Verification items for this drawing (mm, ordinates from the low corner). A direction names the side the tool comes from. Round coordinates to 2 decimals unless told otherwise and drop trailing zeros. Order: outer loops, then holes, each group sorted by start corner. A loop starts at its lowest first (then second) coordinate and runs counter-clockwise, first axis right, second up. Notation, with made-up numbers: M 9.5,-29.5 L 17.5,-29.5 A31 ccw 17.5,-4.5 Z; hole C -21,85 d3. An arc over 180 degrees is marked long. One line per item, written item: value. Start each with the question number.
(1) Release check for a two-part mould opening along Z. For the marked faces 1, 2 and 3 record: released by +Z, released by -Z, zero draft, split by the parting line, or undercut.
(2) Thickness scan on L1, parallel to Y at x = 2.75, z = 67 (1 decimal); L2, parallel to Y at x = 7.75, z = 13.5 (1 decimal); L3, parallel to Z at x = 3.25, y = 56.5 (1 decimal). Record the ranges inside material, lowest first.
(3) Cross-section at C-C, the plane z = 18. Enter the section's corners in (x, y) (1 decimal).
(4) Depth check by flat-ended pin: pin 1 Ø2 at (x, y) = (11.5, 47) entering from +Z; pin 2 Ø1 at (x, z) = (18.5, 51) entering from +Y (1 decimal); pin 3 Ø14 at (y, z) = (15.621, 39.751) entering from +X; pin 4 Ø1 at (x, z) = (10, 40) entering from -Y. Enter the tip coordinate at first touch or a pass-through.
(5) Cross-section at B-B, the plane x = 16.25. Enter the section's corners in (y, z).
(6) Cross-section at D-D, the plane y = 22. Enter the section's corners in (x, z) (1 decimal), and give its area (3 significant figures).
(7) Access from +Z, -Z, +X, -X, +Y, -Y to the whole of each face (thin tool, end or side, straight path). Record for the marked faces 4 and 5.
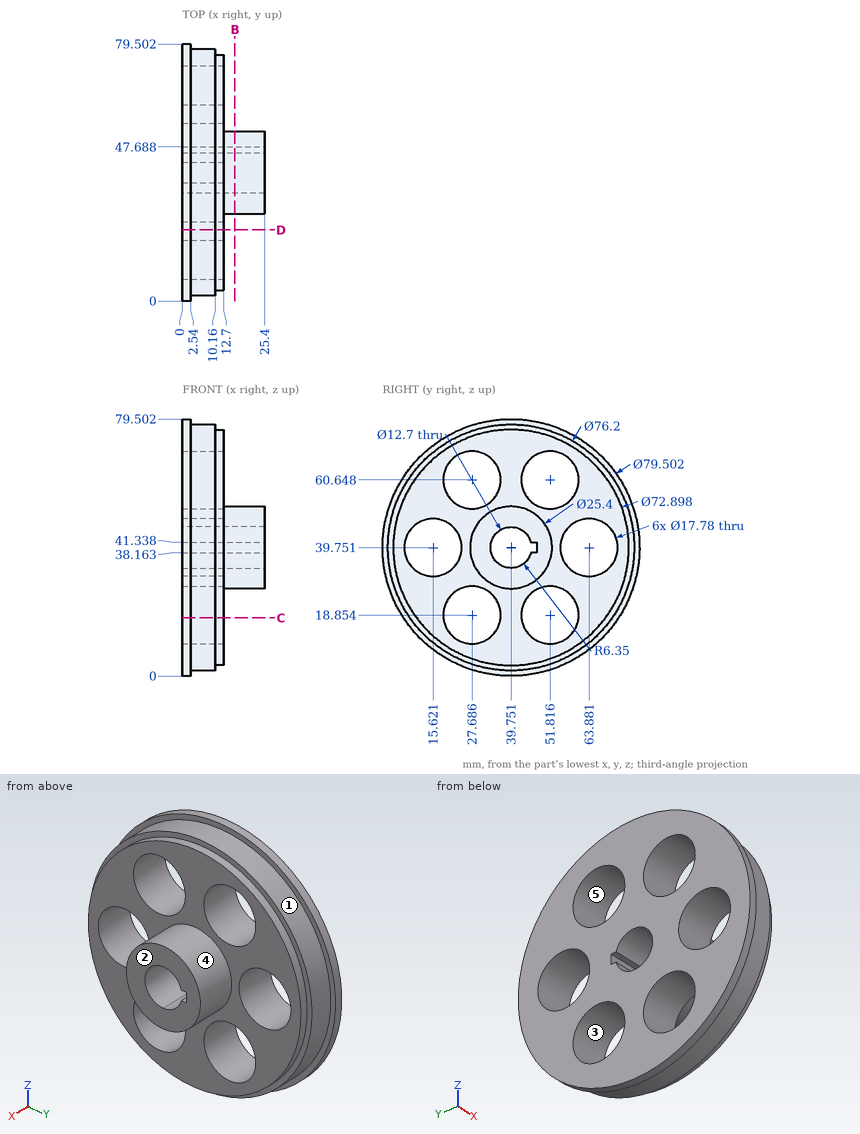
Values found:
1. face 1: split by the parting line
1. face 2: zero draft
1. face 3: undercut
2. L1: 13.1 to 21.5, 33.9 to 45.6, 58 to 66.4
2. L2: 12.1 to 20.6, 34.8 to 44.7, 58.9 to 67.4
2. L3: 5.5 to 11.3, 26.4 to 34.8, 44.7 to 53.1, 68.2 to 74
3. outline: M 0,6.5 L 2.5,6.5 L 2.5,8.5 L 10.2,8.5 L 10.2,10.5 L 12.7,10.5 L 12.7,18.8 L 0,18.8 Z; M 0,36.5 L 12.7,36.5 L 12.7,43 L 0,43 Z; M 0,60.7 L 12.7,60.7 L 12.7,69 L 10.2,69 L 10.2,71 L 2.5,71 L 2.5,73 L 0,73 Z
4. pin 1: z = 75.66
4. pin 2: y = 46.5
4. pin 3: through
4. pin 4: y = 1.65
5. outline: C 39.75,39.75 d25.4; hole M 45.9,38.16 L 47.69,38.16 L 47.69,41.34 L 45.9,41.34 A6.35 ccw long Z
6. outline: M 0,4.2 L 2.5,4.2 L 2.5,6 L 10.2,6 L 10.2,7.9 L 12.7,7.9 L 12.7,12 L 0,12 Z; M 0,25.7 L 12.7,25.7 L 12.7,33.6 L 0,33.6 Z; M 0,45.9 L 12.7,45.9 L 12.7,53.8 L 0,53.8 Z; M 0,67.5 L 12.7,67.5 L 12.7,71.6 L 10.2,71.6 L 10.2,73.5 L 2.5,73.5 L 2.5,75.3 L 0,75.3 Z
6. area: 352 mm^2
7. face 4: +X
7. face 5: +X, -X
